Print and shaded views of the part. All mm, measured from the part's lowest x, y and z. A direction names the side the tool comes from. Give positions to 0.01 mm unless a question says otherwise; leave off trailing zeros. Loops run counter-clockwise (first coordinate to the right, second up) from the corner with the lowest first, then second, coordinate; pieces in that order, holes last. Notation, with made-up numbers: M -31,73 L -7,73 A10 cw -7,86 Z; hole C 31,36 d9. An arc over 180 degrees is marked long. Answer in a Markdown table with one row per item.
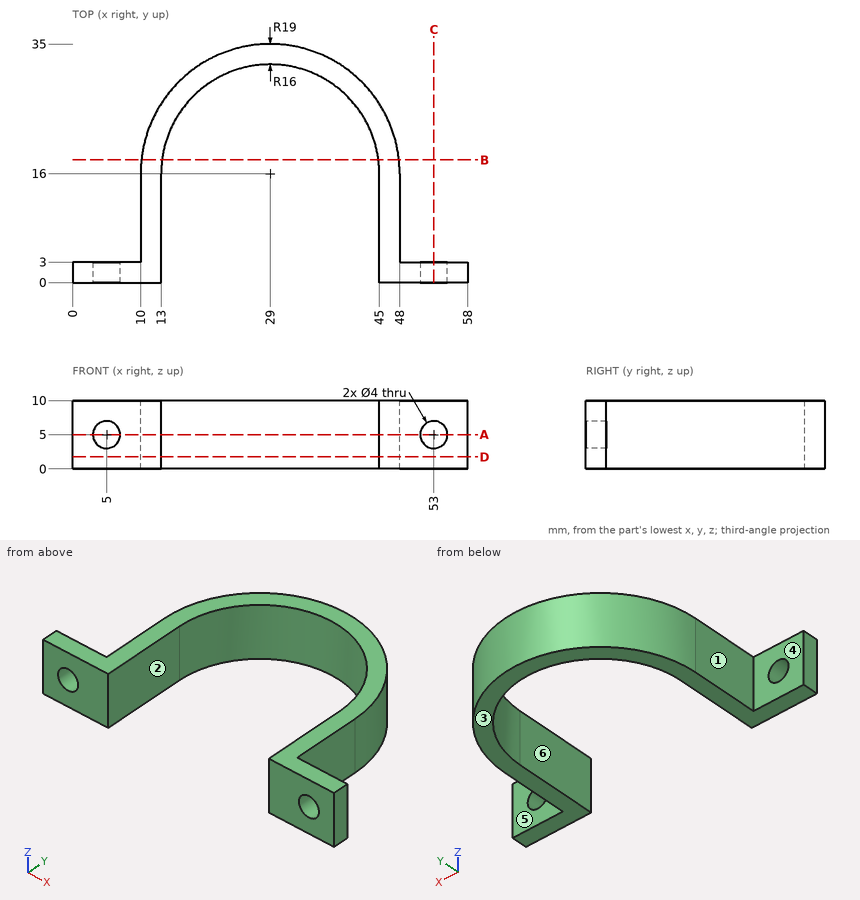
(1) Saw through at C-C, the plane x = 53. Give the cut face in (y, z).
Established:
| item | result |
|---|---|
| outline | M 0,0 L 3,0 L 3,3 L 0,3 Z; M 0,7 L 3,7 L 3,10 L 0,10 Z |
(2) Saw through at D-D, the plane z = 1.75. Give the cut face in (x, y).
Established:
| item | result |
|---|---|
| outline | M 0,0 L 13,0 L 13,16 A16 cw 45,16 L 45,0 L 58,0 L 58,3 L 48,3 L 48,16 A19 ccw 10,16 L 10,3 L 0,3 Z |
(3) Wall check: L1, parallel to Z at x = 53, y = 0.65; L2, parallel to X at y = 14, z = 6; L3, parallel to Y at x = 54.5, z = 9.25. Give the ranges that are in metal, low to high.
Established:
| item | result |
|---|---|
| L1 | z = 0 to 3, 7 to 10 |
| L2 | x = 10 to 13, 45 to 48 |
| L3 | y = 0 to 3 |
(4) Saw through at A-A, the plane z = 5. Give the cut face in (x, y).
Established:
| item | result |
|---|---|
| outline | M 0,0 L 3,0 L 3,3 L 0,3 Z; M 7,0 L 13,0 L 13,16 A16 cw 45,16 L 45,0 L 51,0 L 51,3 L 48,3 L 48,16 A19 ccw 10,16 L 10,3 L 7,3 Z; M 55,0 L 58,0 L 58,3 L 55,3 Z |
(5) Mould opens along X. For the marked faces 1, 2 and 3 say: pulls with the +X half, pulls with the -X half, needs draft (parallel to the pull), parting line crosses it, or undercut.
Established:
| item | result |
|---|---|
| face 1 | pulls with the -X half |
| face 2 | undercut |
| face 3 | needs draft |
(6) Saw through at B-B, the plane y = 18. Give the cut face in (x, z), and give its area (3 significant figures).
Established:
| item | result |
|---|---|
| outline | M 10.11,0 L 13.13,0 L 13.13,10 L 10.11,10 Z; M 44.87,0 L 47.89,0 L 47.89,10 L 44.87,10 Z |
| area | 60.4 mm2 |
(7) Which spindle directions (+Z, -Z, +X, -X, +Y, -Y) get a long thin tool onto all of the face, cutting with end or side? Do the marked faces 4, 5 and 6. Say none if no direction does.
Established:
| item | result |
|---|---|
| face 4 | +Z, -Z, -X, +Y |
| face 5 | +Z, -Z, +X, +Y |
| face 6 | +Z, -Z, -Y |
(8) Flat gauge pins, fed straight in: P1, Ø3, axis at x = 5, z = 5, coming from the -Y side; P2, Ø5, axis at x = 7, z = 6.5, coming from the +Y side; P3, Ø6, axis at y = 12, z = 2, coming from the +X side; P4, Ø3, axis at y = 10, z = 4, coming from the -X side. Where does each tip first touch, or does it go through?
Established:
| item | result |
|---|---|
| P1 | passes through |
| P2 | stops at y = 3 |
| P3 | stops at x = 48 |
| P4 | stops at x = 10 |
